Autodesk Inventor part; units mm, degrees
ref_plane "Work Plane1" through (0, 4.7625, 0) normal (0, 1, 0) x (1, 0, 0)
ref_plane "YZ Plane" through (0, 0, 0) normal (1, 0, 0) x (0, 1, 0)
ref_plane "XZ Plane" through (0, 0, 0) normal (0, 1, 0) x (-1, 0, 0)
sketch "Sketch1" plane through (0, 0, 0) normal (0, 1, 0) x (-1, 0, 0)
  circle A0 centre (0, 0) radius 22.225 construction
  circle A1 centre (0, 0) radius 17.65
  circle A2 centre (0, 0) radius 22.225
  dimension "d0" = 44.45
  dimension "d1" = 35.3
  dimension "d2" = 44.45
extrude "Extrusion1" add sketch "Sketch1" along normal blind 9.525
sketch "Sketch2" plane through (0, 0, 0) normal (0, -1, 0) x (1, 0, 0)
  circle A0 centre (0, 0) radius 17.6
  circle A1 centre (0, 0) radius 20.6375
  dimension "d5" = 41.275
  dimension "d6" = 35.2
extrude "Extrusion2" add sketch "Sketch2" along normal blind 1.5875
sketch "Sketch3" plane through (0, 9.525, 0) normal (0, 1, 0) x (1, 0, 0)
  circle A0 centre (0, 0) radius 17.65
  circle A1 centre (0, 0) radius 20.6375
  dimension "d9" = 35.3
  dimension "d10" = 41.275
extrude "Extrusion3" add sketch "Sketch3" along normal blind 1.5875
sketch "Sketch4" plane through (0, 0, 0) normal (1, 0, 0) x (0, 1, 0)
  line L0 (11.1125, -17.65) -> (17.8875, -17.65)
  line L1 (17.8875, -17.65) -> (17.8875, -20.6375)
  line L2 (17.8875, -20.6375) -> (11.1125, -20.6375) construction
  line L3 (11.1125, -20.6375) -> (11.1125, -17.65)
  line L4 (11.1125, -20.6375) -> (11.1125, 20.6375)
  line L5 (12.7, -17.65) -> (12.7, -20.6375) construction
  line L6 (11.1125, -20.6375) -> (12.7, -19.8438)
  line L7 (12.7, -19.8438) -> (17.8875, -19.8438)
  line L8 (0, 0) -> (25.7056, 0) construction
  line L9 (-11.1125, 0) -> (-11.1125, -19.8438) construction
  line L10 (0, 20.6375) -> (0, -20.6375)
  dimension "d13" = 17.65
  dimension "d14" = 20.6375
  dimension "d16" = 1.5875
  dimension "d18" = 19.8438
  dimension "d84" = 11.1125
  dimension "d85" = 29
revolve "Revolution1" add sketch "Sketch4" angle 360 about axis through (0, 0, 0) along (0, 1, 0)
ref_plane "Work Plane1" through (0, 4.7625, 0) normal (0, 1, 0) x (1, 0, 0)
sketch "Sketch11" plane through (0, 17.8875, 0) normal (0, 1, 0) x (1, 0, 0)
  circle A0 centre (0, 0) radius 11.75 construction
  line L0 (0, 0) -> (-11.75, 0) construction
  circle A1 centre (-11.75, 0) radius 3.875
  line L1 (-11.75, -3.875) -> (-18.1, -3.875)
  line L2 (-18.1, -3.875) -> (-18.1, 3.875)
  line L3 (-18.1, 3.875) -> (-11.75, 3.875)
  line L4 (-11.75, 3.875) -> (-11.75, -3.875) construction
  circle A2 centre (0, -11.75) radius 3.875
  line L5 (3.875, -11.75) -> (3.875, -18.1)
  line L6 (3.875, -18.1) -> (-3.875, -18.1)
  line L7 (-3.875, -18.1) -> (-3.875, -11.75)
  line L8 (-3.875, -11.75) -> (3.875, -11.75) construction
  circle A3 centre (11.75, 0) radius 3.875
  line L9 (11.75, 3.875) -> (18.1, 3.875)
  line L10 (18.1, 3.875) -> (18.1, -3.875)
  line L11 (18.1, -3.875) -> (11.75, -3.875)
  line L12 (11.75, -3.875) -> (11.75, 3.875) construction
  circle A4 centre (0, 11.75) radius 3.875
  line L13 (-3.875, 11.75) -> (-3.875, 18.1)
  line L14 (-3.875, 18.1) -> (3.875, 18.1)
  line L15 (3.875, 18.1) -> (3.875, 11.75)
  line L16 (3.875, 11.75) -> (-3.875, 11.75) construction
  circle A5 centre (0, -11.75) radius 1.7526
  circle A6 centre (11.75, 0) radius 1.7526
  circle A7 centre (0, 11.75) radius 1.7526
  circle A8 centre (-11.75, 0) radius 1.7526
  point P0 (3.875, 11.75)
  point P1 (11.75, -3.875)
  point P2 (-3.875, -11.75)
  point P3 (-11.75, 3.875)
  dimension "d121" = 23.5
  dimension "d122" = 7.75
  dimension "d123" = 6.35
  dimension "d126" = 360
  dimension "d134" = 3.5052
  dimension "d137" = 360
extrude "Extrusion10" add sketch "Sketch11" against normal blind 3
fillet "Fillet5" radius 0.5 8 edges at (-17.2194, 16.3875, -3.875) (-17.2194, 16.3875, 3.875) (-3.875, 16.3875, 17.2194) (3.875, 16.3875, 17.2194) (17.2194, 16.3875, -3.875) (17.2194, 16.3875, 3.875) (-3.875, 16.3875, -17.2194) (3.875, 16.3875, -17.2194)
chamfer "Chamfer5" distance 1.5875 angle 45 1 edges at (-17.6, -1.5875, 0)
chamfer "Chamfer6" distance 1.5875 angle 45 2 edges at (22.225, 9.525, 0) (22.225, 0, 0)
properties part number "Motor Hub" material "Nylon 6/6"
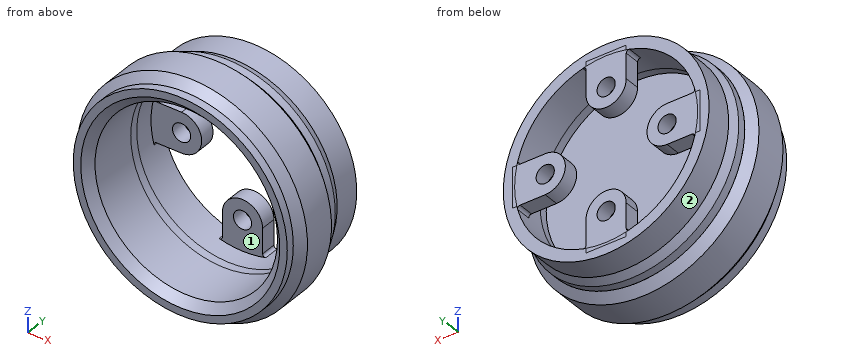
CAD build for the part. Positions are in the model's coordinates, mm. Face numbers are marked on the shaded views. Give positions to 0.01 mm unless a question says otherwise; leave off trailing zeros. Write each loop counter-clockwise with the first axis right and the second up, starting at its lowest first coordinate (ties: lowest second). Pieces come first, ordered by that corner, then holes. Notation, with made-up numbers: M 42,42 L 55,42 A16 ccw 55,56 Z; hole C -23,75 d6. An arc over 180 degrees is marked long. Return JSON: item names as keys, results as strings. Group by question number.
(1) Flat gauge pins, fed straight in: pin 1 Ø3.5 at (x, y) = (-15, 16) entering from +Z; pin 2 Ø0.9 at (y, z) = (17, 15.5) entering from +X; pin 3 Ø8 at (y, z) = (13.5, -11) entering from +X. Where does each tip first touch, or does it go through?
(2) Mould opens along X. For the marked faces 1 and 2 say: pulls with the +X half, pulls with the -X half, needs draft (parallel to the pull), parting line crosses it, or undercut.
(3) Band-saw the part on B-B (x = 0). State how many separate pieces and enclosed holes the cut face has, and give its area (3 significant figures).
(4) Drill centre lines: L1, parallel to Z at x = 0, y = 16.8 (3 decimals); L2, parallel to Z at x = -11.75, y = 16.75 (3 decimals); L3, parallel to Z at x = 0, y = 4.5 (3 decimals). Where is each one in solid material? Low to high. Write a range as [from, to].
(5) Band-saw the part on A-A (y = 5.25). Give the cut face in (x, z) (3 decimals).
Entries:
{
 "1": {"pin 1": "stops at z = 14.77", "pin 2": "stops at x = 12.93", "pin 3": "stops at x = 19.11"},
 "2": {"face 1": "undercut", "face 2": "parting line crosses it"},
 "3": {"separate pieces": "4", "enclosed holes": "0", "area": "167 mm^2"},
 "4": {"L1": "z = [-19.844, -13.503], [-9.997, -7.875], [7.875, 9.997], [13.503, 19.844]", "L2": "z = [-15.991, -13.17], [-3.875, -1.753], [1.753, 3.875], [13.17, 15.991]", "L3": "z = [-22.225, -17.65], [17.65, 22.225]"},
 "5": {"outline": "C 0,0 d44.45; hole C 0,0 d35.3"}
}
